Geometry: final body of the model. Coordinates: model frame, mm. A direction names the side the tool comes from. Give positions to 0.01 mm unless a question says otherwise; leave off trailing zeros. Write each loop counter-clockwise with the first axis right and the second up, starting at its lowest first coordinate (ties: lowest second). Pieces come first, ordered by that corner, then holes. Notation, with made-up numbers: (65, 40.5) -> (100, 40.5) arc R17 cw to (100, 70.5) -> close; hole circle Ø1 at (26.25, 84). An arc over 180 degrees is marked (long way). Answer as a JSON object with one key per item and string values. Group by question number.
(1) Draft query along X for faces 3 (the face through (2, -493, 25)), 4 (the face through (25, -494, 0)), 5 (the face through (0, -493, 25)). Return one class per face: +X half, -X half, draft (parallel to the pull), parting line (faces both ways), or undercut.
(2) Material intervals for probe 1 along Z at (x, y) = (41, -733); probe 2 along Z at (x, y) = (15.5, -41.5), sorted ascending.
(3) Section query C-C on y = -839.5. Output: boundary loops of the cut face in (x, z).
(4) Set-up query: faces 1 (the face through (25, -493, 50)), 2 (the face through (48, -493, 25)). Return all of +Z, -Z, +X, -X, +Y, -Y with unobstructed straight access to the full face (end or side cutting, diameter ignored); none if empty.
(5) Section query A-A on z = 37.5. Output: boundary loops of the cut face in (x, y).
(6) Section query B-B on x = 19.5. Output: boundary loops of the cut face in (y, z).
from build123d import *

# Parameters (mm, degrees)
F0_W     = 50
F0_H     = 50
F0_W_2   = 46
F0_H_2   = 46
F1_DEPTH = 1000
F3_DEPTH = 50.001


# Not quite as in the source:
# - a pattern or mirror of a feature is missing from the dataset's text; its kind, count and spacing are read off the source's solid


with BuildPart() as f1:
    # F0 (on Front) → F1 (new body)
    with BuildSketch(Plane.XZ):
        with Locations((25, 25)):
            Rectangle(F0_W, F0_H)
        with Locations((25, 25)):
            Rectangle(F0_W_2, F0_H_2, mode=Mode.SUBTRACT)
    extrude(amount=F1_DEPTH)

    # F2 (on face) → F3 (cut, through all)
    with BuildSketch(Plane.YZ.offset(50)):
        Polygon((-950, 0), (-1000, 50), (-1000, 0), align=None)
    f3 = extrude(amount=-F3_DEPTH, mode=Mode.SUBTRACT)

    # F3_copies: F3 across plane
    add(f3.mirror(Plane.ZX.offset(-500)), mode=Mode.SUBTRACT)


solid = f1.part
Answer list:
{
 "1": {"face 3": "undercut", "face 4": "draft", "face 5": "-X half"},
 "2": {"probe 1": "0 to 2, 48 to 50", "probe 2": "48 to 50"},
 "3": {"outline": "(0, 0) -> (50, 0) -> (50, 50) -> (0, 50) -> close; hole (2, 2) -> (48, 2) -> (48, 48) -> (2, 48) -> close"},
 "4": {"face 1": "+Z, +X, -X, +Y, -Y", "face 2": "+Y, -Y"},
 "5": {"outline": "(0, -987.5) -> (2, -987.5) -> (2, -12.5) -> (0, -12.5) -> close; (48, -987.5) -> (50, -987.5) -> (50, -12.5) -> (48, -12.5) -> close"},
 "6": {"outline": "(-1000, 50) -> (-998, 48) -> (-2, 48) -> (0, 50) -> close; (-952, 2) -> (-950, 0) -> (-50, 0) -> (-48, 2) -> close"}
}
